from build123d import *

# Parameters (mm, degrees)
SKETCH1_R           = 10
BOSS_EXTRUDE1_DEPTH = 1
SKETCH2_R           = 10
BOSS_EXTRUDE2_DEPTH = 4
SKETCH4_R           = 13
BOSS_EXTRUDE3_DEPTH = 1
CUT_SWEEP1_START    = 4.993438222
CUT_SWEEP1_DEPTH    = 4.55597903
SKETCH9_R           = 2.5
CUT_EXTRUDE2_DEPTH  = 5
SKETCH10_R          = 2.5
SKETCH10_R_2        = 1
BOSS_EXTRUDE4_DEPTH = 1
SKETCH11_R          = 13
SKETCH11_R_2        = 10
BOSS_EXTRUDE5_DEPTH = 1


# Read off the part's stored shape, not the designer's step: Cut-Sweep1
with BuildPart() as part:
    # Sketch1 → Boss-Extrude1 (new body)
    with BuildSketch(Plane(origin=(0, 0, 0), x_dir=(1, 0, 0), z_dir=(0, 1, 0))):
        with Locations(Location((0, 0, 0), (0, 0, 270))):
            Circle(SKETCH1_R)
    extrude(amount=BOSS_EXTRUDE1_DEPTH)

    # Sketch2 → Boss-Extrude2 (add)
    with BuildSketch(Plane(origin=(0, 0, 0), x_dir=(1, 0, 0), z_dir=(0, 1, 0))):
        with Locations(Location((0, 0, 0), (0, 0, 270))):
            Circle(SKETCH2_R)
    extrude(amount=BOSS_EXTRUDE2_DEPTH)

    # Sketch4 → Boss-Extrude3 (add)
    with BuildSketch(Plane(origin=(0, 4, 0), x_dir=(1, 0, 0), z_dir=(0, 1, 0))):
        with Locations(Location((0, 0, 0), (0, 0, 270))):
            Circle(SKETCH4_R)
    extrude(amount=BOSS_EXTRUDE3_DEPTH)

    # Cut-Sweep1 outline → Cut-Sweep1 (cut)
    with BuildSketch(Plane(origin=(0, 0, 0), x_dir=(1, 0, 0), z_dir=(0, 0.6401843996644766, 0.7682212795973786)).offset(CUT_SWEEP1_START)):
        with BuildLine():
            add(Edge.make_bspline(
                [(0, -4.801382997), (1, -4.801382997), (1, -4.161198598), (0, -4.161198598), (-1, -4.161198598), (-1, -4.801382997), (0, -4.801382997)],
                knots=[0, 0, 0, 0, 0.5, 0.5, 0.5, 1, 1, 1, 1], degree=3, weights=[1, 0.333333333, 0.333333333, 1, 0.333333333, 0.333333333, 1]))
        make_face()
    extrude(amount=CUT_SWEEP1_DEPTH, mode=Mode.SUBTRACT)

    # Sketch9 → Cut-Extrude2 (cut)
    with BuildSketch(Plane(origin=(0, 0, 0), x_dir=(1, 0, 0), z_dir=(0, 1, 0))):
        with Locations(Location((0, 0, 0), (0, 0, 270))):
            Circle(SKETCH9_R)
    extrude(amount=CUT_EXTRUDE2_DEPTH, mode=Mode.SUBTRACT)

    # Sketch10 → Boss-Extrude4 (add)
    with BuildSketch(Plane(origin=(0, 0, 0), x_dir=(1, 0, 0), z_dir=(0, 1, 0))):
        with Locations(Location((0, 0, 0), (0, 0, 270))):
            Circle(SKETCH10_R)
        with Locations(Location((0, 0, 0), (0, 0, 270))):
            Circle(SKETCH10_R_2, mode=Mode.SUBTRACT)
    extrude(amount=BOSS_EXTRUDE4_DEPTH)

    # Sketch11 → Boss-Extrude5 (add)
    with BuildSketch(Plane(origin=(0, 0, 0), x_dir=(-1, 0, 0), z_dir=(0, -1, 0))):
        with Locations(Location((0, 0, 0), (0, 0, 270))):
            Circle(SKETCH11_R)
        with Locations(Location((0, 0, 0), (0, 0, 90))):
            Circle(SKETCH11_R_2, mode=Mode.SUBTRACT)
    extrude(amount=-BOSS_EXTRUDE5_DEPTH)


solid = part.part
Model file for the job. Use its own axes, mm. A direction names the side the tool comes from. Give positions to 0.01 mm unless a question says otherwise; leave off trailing zeros. Order: outer loops, then holes, each group sorted by start corner. A loop starts at its lowest first (then second) coordinate and runs counter-clockwise, first axis right, second up. Notation, with made-up numbers: M 28.5,34.5 L 36.5,34.5 A26 ccw 36.5,70.5 Z; hole C 64.5,-11.5 d8. An arc over 180 degrees is marked long. Put each result on its own line as item: value. Start each with the question number.
(1) Pin check, flat tips, straight feed: pin 1 Ø4 at (x, z) = (-0.5, -0.5) entering from +Y; pin 2 Ø1.2 at (x, z) = (0, 0) entering from -Y; pin 3 Ø1.5 at (y, z) = (2.5, -4) entering from +X; pin 4 Ø1 at (x, y) = (8, 4) entering from -Z. Stop position of each tip, or through.
(2) Pull direction X, two halves, no side cores. Call faces 1 (the face through (0, 5, 3)), 2 (the face through (-7.91, 4.493, -10.316)), 3 (the face through (-0.976, 0.493, -0.217)): released by +X, released by -X, zero draft, split by the parting line, or undercut.
(3) Band-saw the part on A-A on z = 0. Give the cut face in (x, y).
(4) Band-saw the part on B-B on x = 11.5. Give the cut face in (y, z), then the cut area to 3 significant figures.
(5) Tool access for faces 4 (the face through (7.91, 0.493, -10.316)), 5 (the face through (8, 1, 7)), 6 (the face through (-2.44, 2.97, -0.54)): list every direction of +Z, -Z, +X, -X, +Y, -Y with a clear straight run to the whole face (end or side of a thin tool).
(6) Band-saw the part on D-D on x = 8. Give the cut face in (y, z).
(7) Drill centre lines: L1, parallel to Y at x = 9.5, z = -7.5; L2, parallel to X at y = 3.6, z = 0; L3, parallel to Y at x = -1.25, z = -1.75. Where is each one in solid material? Low to high. Write a range as [from, to].
(8) Band-saw the part on C-C on y = 3.4. Give the cut face in (x, z), then the cut area to 3 significant figures.
Results below:
1. pin 1: stops at y = 5
1. pin 2: passes through
1. pin 3: stops at x = 9.46
1. pin 4: stops at z = -10.62
2. face 1: zero draft
2. face 2: split by the parting line
2. face 3: undercut
3. outline: M -13,0 L -1,0 L -1,1 L -2.5,1 L -2.5,5 L -13,5 L -13,4 L -10,4 L -10,1 L -13,1 Z; M 1,0 L 13,0 L 13,1 L 10,1 L 10,4 L 13,4 L 13,5 L 2.5,5 L 2.5,1 L 1,1 Z
4. outline: M 0,-6.06 L 1,-6.06 L 1,6.06 L 0,6.06 Z; M 4,-6.06 L 5,-6.06 L 5,6.06 L 4,6.06 Z
4. area: 24.2 mm2
5. face 4: +Y, -Y
5. face 5: none
5. face 6: +Y
6. outline: M 0,-10.25 L 1,-10.25 L 1,-6 L 4,-6 L 4,-10.25 L 5,-10.25 L 5,10.25 L 4,10.25 L 4,6 L 1,6 L 1,10.25 L 0,10.25 Z
7. L1: y = [0, 1], [4, 5]
7. L2: x = [-10, -2.5], [2.5, 10]
7. L3: y = [0, 1]
8. outline: C 0,0 d20; hole C 0,0 d5
8. area: 295 mm2
